Build history of the part. All positions in model axes, mm. Face numbers are marked on the shaded views. Give positions to 0.01 mm unless a question says otherwise; leave off trailing zeros. Write each loop counter-clockwise with the first axis right and the second up, starting at its lowest first coordinate (ties: lowest second). Pieces come first, ordered by that corner, then holes. Notation, with made-up numbers: M -26,0.5 L 15,0.5 A16 cw 15,27.5 Z; hole C 52,21 d1. An arc over 180 degrees is marked long. Return JSON: item names as keys, results as strings. Group by question number.
Q1. Band-saw the part on C-C, the plane z = 0.5. Give the cut face in (x, y) (3 decimals), then the cut area to 3 significant figures.
Q2. Wall check: probe 1 along Y at (x, z) = (0, -3) (3 decimals); probe 2 along Y at (x, z) = (2.5, -0.5); probe 3 along Y at (x, z) = (-2.75, 3.25). Give the ranges that are in metal, low to high.
Q3. Pull direction Y, two halves, no side cores. Call the marked faces 1 and 2: +Y half, -Y half, draft (parallel to the pull), parting line (faces both ways), or undercut.
Q4. Flat gauge pins, fed straight in: pin 1 Ø3 at (x, y) = (1, -25) entering from +Z (3 decimals); pin 2 Ø1.5 at (y, z) = (72, -2.5) entering from +X; pin 3 Ø1 at (x, y) = (1, 43.5) entering from +Z. Where does each tip first touch, or does it go through?
Q5. Band-saw the part on A-A, the plane x = 0. Give the cut face in (y, z) (3 decimals).
Q6. Band-saw the part on B-B, the plane y = 92.5. Give the cut face in (x, z) (3 decimals).
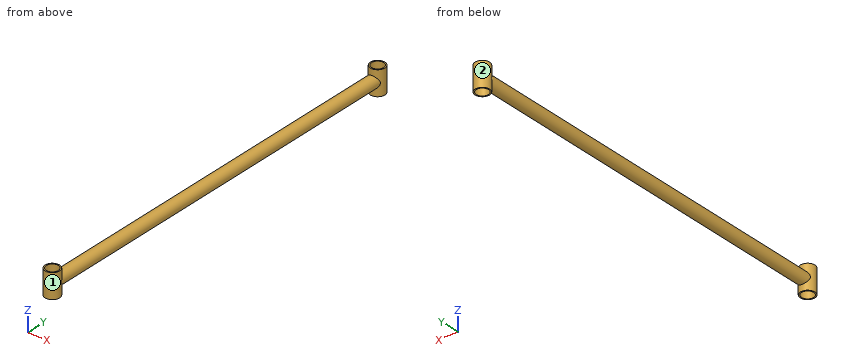
from build123d import *

# Parameters (mm, degrees)
SKETCH3_R           = 3.175
BOSS_EXTRUDE1_DEPTH = 104.775
SKETCH4_R           = 3.81
BOSS_EXTRUDE2_DEPTH = 6.35
SKETCH5_R           = 3.175
CUT_EXTRUDE1_DEPTH  = 12.7


with BuildPart() as part:
    # Sketch3 → Boss-Extrude1 (new, symmetric)
    with BuildSketch(Plane(origin=(0, 0, 0), x_dir=(1, 0, 0), z_dir=(0, 1, 0))):
        with Locations(Location((0, 0, 0), (0, 0, 270))):
            Circle(SKETCH3_R)
    extrude(amount=BOSS_EXTRUDE1_DEPTH, both=True)

    # Sketch4 → Boss-Extrude2 (add, symmetric)
    with BuildSketch(Plane.XY):
        with Locations((0, 104.775)):
            Circle(SKETCH4_R)
    boss_extrude2 = extrude(amount=BOSS_EXTRUDE2_DEPTH, both=True)

    # Sketch5 → Cut-Extrude1 (cut)
    with BuildSketch(Plane.XY.offset(6.35)):
        with Locations((0, 104.775)):
            Circle(SKETCH5_R)
    cut_extrude1 = extrude(amount=-CUT_EXTRUDE1_DEPTH, mode=Mode.SUBTRACT)

    # Mirror1: Boss-Extrude2, Cut-Extrude1 across plane
    add(boss_extrude2.mirror(Plane.ZX))
    add(cut_extrude1.mirror(Plane.ZX), mode=Mode.SUBTRACT)


solid = part.part
From the geometry:
{
 "1": {"outline": "M -3.135,-102.61 A3.81 ccw long 3.135,-102.61 L 3.135,102.61 A3.81 ccw long -3.135,102.61 Z; hole C 0,-104.775 d6.35; hole C 0,104.775 d6.35", "area": "1,300 mm^2"},
 "2": {"probe 1": "y = -108.585 to -107.95, -101.6 to 101.6, 107.95 to 108.585", "probe 2": "y = -107.65 to -106.73, -102.82 to 102.82, 106.73 to 107.65", "probe 3": "y = -107.41 to -106.36, -103.19 to -102.14, 102.14 to 103.19, 106.36 to 107.41"},
 "3": {"face 1": "undercut", "face 2": "undercut"},
 "4": {"pin 1": "stops at z = 3.175", "pin 2": "stops at x = 2.65", "pin 3": "stops at z = 3.14"},
 "5": {"outline": "M -108.585,-6.35 L -107.95,-6.35 L -107.95,6.35 L -108.585,6.35 Z; M -101.6,-6.35 L -100.965,-6.35 L -100.965,-3.175 L 100.965,-3.175 L 100.965,-6.35 L 101.6,-6.35 L 101.6,6.35 L 100.965,6.35 L 100.965,3.175 L -100.965,3.175 L -100.965,6.35 L -101.6,6.35 Z; M 107.95,-6.35 L 108.585,-6.35 L 108.585,6.35 L 107.95,6.35 Z"},
 "6": {"outline": "C 0,0 d6.35"}
}
